Part model, mm, in its own coordinate system. Face numbers are marked on the shaded views. Coordinates: 2 decimals unless noted, no trailing zeros. Loops run counter-clockwise (first coordinate to the right, second up) from the corner with the lowest first, then second, coordinate; pieces in that order, holes last. Notation, with made-up numbers: (37.25, 33.5) - (47.25, 33.5) arc R21 ccw to (47.25, 58.5) - close; hole circle Ø5 at (11, 10.5). An arc over 180 degrees is marked (long way). Use a Markdown table: item, result. Add a question column.
1. Band-saw the part on C-C, the plane y = -3.55. Give the cut face in (x, z).
2. Drop flat-ended pins along their axis: pin 1 (1.1 mm diameter, centred on x = 22, y = -0.5, fed in from +Z); pin 2 (5 mm diameter, centred on x = 121.2, z = -6, fed in from -Y); pin 3 (6 mm diameter, centred on x = 29, z = -25.5, fed in from +Y). Give the stop position or say it passes through.
3. Band-saw the part on B-B, the plane z = -26.5. Give the cut face in (x, y).
4. Pull direction Z, two halves, no side cores. Call the marked faces 1 and 2: pulls with the +Z half, pulls with the -Z half, needs draft (parallel to the pull), parting line crosses it, or undercut.
5. Wall check: probe 1 along X at (y, z) = (-1.8, -6); probe 2 along Z at (x, y) = (6, -3); probe 3 along X at (y, z) = (-3.4, -22.5). Give the ranges that are in metal, low to high. Write a range as [from, to].
6. Band-saw the part on D-D, the plane x = 21.5. Give the cut face in (y, z).
7. Band-saw the part on A-A, the plane x = 114.5. Give the cut face in (y, z).
Autodesk Inventor part; units mm, degrees
ref_plane "YZ Plane" through (0, 0, 0) normal (1, 0, 0) x (0, 1, 0)
ref_plane "XZ Plane" through (0, 0, 0) normal (0, 1, 0) x (-1, 0, 0)
ref_plane "XY Plane" through (0, 0, 0) normal (0, 0, 1) x (1, 0, 0)
sketch "Esboço1" plane through (0, 0, 0) normal (0, 1, 0) x (-1, 0, 0)
  line L0 (0, 0) -> (-127, 0)
  line L1 (-127, 0) -> (-127, -51)
  line L2 (-127, -51) -> (0, -51)
  line L3 (0, -51) -> (0, 0)
  dimension "d0" = 127
  dimension "d1" = 51
extrude "Extrusão1" add sketch "Esboço1" against normal blind 6
sketch "Esboço2" plane through (0, 0, 0) normal (0, 1, 0) x (1, 0, 0)
  line L0 (127, 51) -> (127, 0)
  line L1 (63.5, 0) -> (6, 0)
  line L2 (0, 51) -> (127, 51)
  line L3 (0, 6) -> (6, 6)
  point P0 (6, 45)
  point P1 (121.2, 45)
  point P2 (121.2, 6)
  dimension "d4" = 57.5
hole "Furo1" at (6, 0, -6) at (6, 0, -45) at (121.2, 0, -45) at (121.2, 0, -6) direction (0, -1, 0) diameter 6 end through all
sketch "Esboço3" plane through (0, 0, 0) normal (0, 1, 0) x (1, 0, 0)
  line L0 (127, 0) -> (0, 0)
  line L1 (0, 0) -> (57.5, 0)
  line L2 (0, 51) -> (127, 51)
  line L3 (0, 0) -> (0, 51)
  line L4 (0, 25.5) -> (127, 25.5)
  line L5 (127, 51) -> (127, 0)
  line L6 (0, 25.5) -> (63.5, 25.5)
  circle A0 centre (63.5, 25.5) radius 9.5
  point P0 (57.5, 25.5)
  dimension "d17" = 57.5
  dimension "d47" = 63.5
  dimension "d48" = 19
hole "Furo2" at (63.5, 0, -25.5) direction (0, -1, 0) diameter 19 end through all
sketch "Esboço4" plane through (0, 0, 0) normal (0, 1, 0) x (1, 0, 0)
  line L0 (0, 0) -> (0, 51)
  line L1 (0, 31.5) -> (56.1345, 31.5)
  line L2 (0, 19.5) -> (56.1345, 19.5)
  circle A0 centre (63.5, 25.5) radius 9.5
  circle A1 centre (63.5, 25.5) radius 9.5
extrude "Extrusão2" cut sketch "Esboço4" against normal blind 1 contours L0 L1 A0 L2
sketch "Esboço5" plane through (0, -1, 0) normal (0, 1, 0) x (1, 0, 0)
  circle A0 centre (63.5, 25.5) radius 9.5
  circle A1 centre (63.5, 25.5) radius 9.5
  line L0 (63.5, 25.5) -> (12.5, 25.5)
  point P0 (0, 0)
  dimension "d49" = 51
hole "Furo3" at (12.5, -1, -25.5) direction (0, -1, 0) diameter 4.917 end through all
fillet "Arredondamento1" radius 6 4 edges at (127, -3, -51) (127, -3, 0) (0, -3, 0) (0, -3, -51)
fillet "Arredondamento2" radius 0.5 9 edges at (1.7574, 0, -49.2426) (0, 0, -38.25) (125.2426, 0, -49.2426) (127, 0, -25.5) (125.2426, 0, -1.7574) (63.5, 0, 0) (1.7574, 0, -1.7574) (0, 0, -12.75) (63.5, 0, -51)
sketch "Esboço6" plane through (0, 0, 0) normal (0, 1, 0) x (1, 0, 0)
  circle A0 centre (12.5, 25.5) radius 2.4585
  circle A1 centre (12.5, 25.5) radius 2.4585
  line L0 (12.5, 25.5) -> (114.5, 25.5)
  point P0 (0, 0)
  dimension "d50" = 102
hole "Furo4" at (114.5, 0, -25.5) direction (0, -1, 0) diameter 4.917 end through all
sketch "Sketch7" plane through (0, -6, 0) normal (0, -1, 0) x (1, 0, 0)
  point P0 (12.5, -25.5)
hole "Hole5" at (12.5, -6, -25.5) direction (0, 1, 0) diameter 6.6 end through all
properties part number "base_plate" material "Aluminum 6061-AHC"
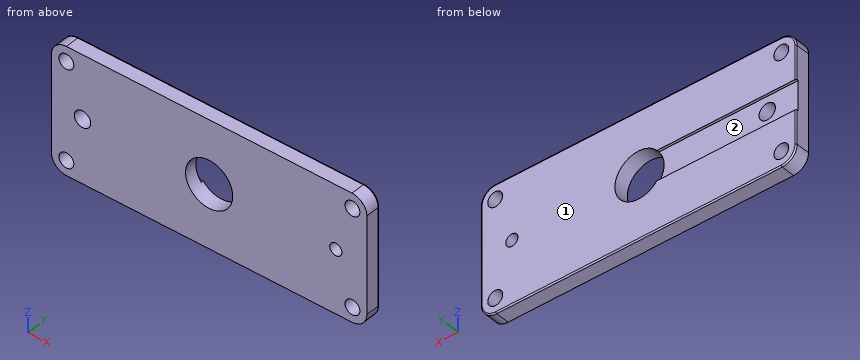
Geometry check:
| question | item | result |
|---|---|---|
| 1 | outline | (0, -45) arc R6 ccw to (6, -51) - (121, -51) arc R6 ccw to (127, -45) - (127, -6) arc R6 ccw to (121, 0) - (6, 0) arc R6 ccw to (0, -6) - close; hole circle Ø6 at (6, -45); hole circle Ø6 at (6, -6); hole circle Ø6.6 at (12.5, -25.5); hole circle Ø19 at (63.5, -25.5); hole circle Ø4.92 at (114.5, -25.5); hole circle Ø6 at (121.2, -45); hole circle Ø6 at (121.2, -6) |
| 2 | pin 1 | stops at z = 0 |
| 2 | pin 2 | passes through |
| 2 | pin 3 | stops at y = -1 |
| 3 | outline | (0, -6) - (9.36, -6) - (9.36, -1) - (0, -1) - close; (15.64, -6) - (54.05, -6) - (54.05, -1) - (15.64, -1) - close; (72.95, -6) - (112.25, -6) - (112.25, 0) - (72.95, 0) - close; (116.75, -6) - (127, -6) - (127, -0.5) arc R0.5 ccw to (126.5, 0) - (116.75, 0) - close |
| 4 | face 1 | needs draft |
| 4 | face 2 | undercut |
| 5 | probe 1 | x = [0, 3], [9, 118.2], [124.2, 127] |
| 5 | probe 2 | z = [-51, -48], [-42, -9], [-3, 0] |
| 5 | probe 3 | x = [0, 11.13], [13.87, 54.49], [72.51, 127] |
| 6 | outline | (-6, -51) - (-0.5, -51) arc R0.5 ccw to (0, -50.5) - (0, -31.5) - (-1, -31.5) - (-1, -19.5) - (0, -19.5) - (0, -0.5) arc R0.5 ccw to (-0.5, 0) - (-6, 0) - close |
| 7 | outline | (-6, -51) - (-0.5, -51) arc R0.5 ccw to (0, -50.5) - (0, -27.96) - (-6, -27.96) - close; (-6, -23.04) - (0, -23.04) - (0, -0.5) arc R0.5 ccw to (-0.5, 0) - (-6, 0) - close |
